from build123d import *

# Parameters (mm, degrees)
SKETCH1_R           = 70
BOSS_EXTRUDE2_DEPTH = 25
SKETCH3_R           = 70
BOSS_EXTRUDE3_DEPTH = 10
SKETCH4_R           = 3
CUT_EXTRUDE1_DEPTH  = 4
SKETCH5_R           = 23.5
CUT_EXTRUDE2_DEPTH  = 7
SKETCH6_R           = 1.5
CUT_EXTRUDE3_DEPTH  = 7
SKETCH7_R           = 22
CUT_EXTRUDE4_DEPTH  = 7
SKETCH8_R           = 70
CUT_EXTRUDE5_DEPTH  = 3
SKETCH9_R           = 1.425
CUT_EXTRUDE6_DEPTH  = 20


with BuildPart() as part:
    # Sketch1 → Boss-Extrude2 (new body)
    with BuildSketch(Plane.XY):
        Circle(SKETCH1_R)
        with BuildLine():
            ThreePointArc((5.084181722, 54.049826689), (0, 56.5), (-5.084181722, 54.049826689))
            ThreePointArc((-5.084181722, 54.049826689), (-14.092268161, 47.993857843), (-24.944456649, 48.218323814))
            ThreePointArc((-24.944456649, 48.218323814), (-30.546206186, 47.530824605), (-33.49862832, 42.720891489))
            ThreePointArc((-33.49862832, 42.720891489), (-37.802608913, 32.756147086), (-47.053406284, 27.077843822))
            ThreePointArc((-47.053406284, 27.077843822), (-51.394207738, 23.470948235), (-51.277497116, 17.828375092))
            ThreePointArc((-51.277497116, 17.828375092), (-49.510888436, 7.118591073), (-54.223231887, -2.659660261))
            ThreePointArc((-54.223231887, -2.659660261), (-55.924911466, -8.040788362), (-52.776122888, -12.724524427))
            ThreePointArc((-52.776122888, -12.724524427), (-45.499810707, -20.779067307), (-44.177564489, -31.552741003))
            ThreePointArc((-44.177564489, -31.552741003), (-42.699850951, -36.999631468), (-37.51870254, -39.237477348))
            ThreePointArc((-37.51870254, -39.237477348), (-27.042864565, -42.079518636), (-20.105832509, -50.428049418))
            ThreePointArc((-20.105832509, -50.428049418), (-15.917889462, -54.211353009), (-10.349359231, -53.29280845))
            ThreePointArc((-10.349359231, -53.29280845), (0, -50.020020118), (10.349359231, -53.29280845))
            ThreePointArc((10.349359231, -53.29280845), (15.917889462, -54.211353009), (20.105832509, -50.428049418))
            ThreePointArc((20.105832509, -50.428049418), (27.042864565, -42.079518636), (37.51870254, -39.237477348))
            ThreePointArc((37.51870254, -39.237477348), (42.699850951, -36.999631468), (44.177564489, -31.552741003))
            ThreePointArc((44.177564489, -31.552741003), (45.499810707, -20.779067307), (52.776122888, -12.724524427))
            ThreePointArc((52.776122888, -12.724524427), (55.924911466, -8.040788362), (54.223231887, -2.659660261))
            ThreePointArc((54.223231887, -2.659660261), (49.510888436, 7.118591073), (51.277497116, 17.828375092))
            ThreePointArc((51.277497116, 17.828375092), (51.394207738, 23.470948235), (47.053406284, 27.077843822))
            ThreePointArc((47.053406284, 27.077843822), (37.802608913, 32.756147086), (33.49862832, 42.720891489))
            ThreePointArc((33.49862832, 42.720891489), (30.546206186, 47.530824605), (24.944456649, 48.218323814))
            ThreePointArc((24.944456649, 48.218323814), (14.092268161, 47.993857843), (5.084181722, 54.049826689))
        make_face(mode=Mode.SUBTRACT)
    extrude(amount=BOSS_EXTRUDE2_DEPTH)

    # Sketch3 → Boss-Extrude3 (add)
    with BuildSketch(Plane.XY.offset(25)):
        Circle(SKETCH3_R)
    extrude(amount=BOSS_EXTRUDE3_DEPTH)

    # Sketch4 → Cut-Extrude1 (cut)
    with BuildSketch(Plane(origin=(0, 0, 25), x_dir=(-1, 0, 0), z_dir=(0, 0, -1))):
        with Locations((0, 50)):
            Circle(SKETCH4_R)
        with Locations((27.032040873, 42.062676642)):
            Circle(SKETCH4_R)
        with Locations((45.481599768, 20.77075065)):
            Circle(SKETCH4_R)
        with Locations((49.491072094, -7.115741914)):
            Circle(SKETCH4_R)
        with Locations((37.787478718, -32.743036697)):
            Circle(SKETCH4_R)
        with Locations((14.086627842, -47.974648681)):
            Circle(SKETCH4_R)
        with Locations((-14.086627842, -47.974648681)):
            Circle(SKETCH4_R)
        with Locations((-37.787478718, -32.743036697)):
            Circle(SKETCH4_R)
        with Locations((-49.491072094, -7.115741914)):
            Circle(SKETCH4_R)
        with Locations((-45.481599768, 20.77075065)):
            Circle(SKETCH4_R)
        with Locations((-27.032040873, 42.062676642)):
            Circle(SKETCH4_R)
    extrude(amount=-CUT_EXTRUDE1_DEPTH, mode=Mode.SUBTRACT)

    # Sketch5 → Cut-Extrude2 (cut)
    with BuildSketch(Plane(origin=(0, 0, 25), x_dir=(-1, 0, 0), z_dir=(0, 0, -1))):
        Circle(SKETCH5_R)
    extrude(amount=-CUT_EXTRUDE2_DEPTH, mode=Mode.SUBTRACT)

    # Sketch6 → Cut-Extrude3 (cut)
    with BuildSketch(Plane(origin=(0, 0, 29), x_dir=(-1, 0, 0), z_dir=(0, 0, -1))):
        with Locations((0, 50)):
            Circle(SKETCH6_R)
        with Locations((27.032040873, 42.062676642)):
            Circle(SKETCH6_R)
        with Locations((45.481599768, 20.77075065)):
            Circle(SKETCH6_R)
        with Locations((49.491072094, -7.115741914)):
            Circle(SKETCH6_R)
        with Locations((37.787478718, -32.743036697)):
            Circle(SKETCH6_R)
        with Locations((14.086627842, -47.974648681)):
            Circle(SKETCH6_R)
        with Locations((-14.086627842, -47.974648681)):
            Circle(SKETCH6_R)
        with Locations((-37.787478718, -32.743036697)):
            Circle(SKETCH6_R)
        with Locations((-49.491072094, -7.115741914)):
            Circle(SKETCH6_R)
        with Locations((-45.481599768, 20.77075065)):
            Circle(SKETCH6_R)
        with Locations((-27.032040873, 42.062676642)):
            Circle(SKETCH6_R)
    extrude(amount=-CUT_EXTRUDE3_DEPTH, mode=Mode.SUBTRACT)

    # Sketch7 → Cut-Extrude4 (cut)
    with BuildSketch(Plane(origin=(0, 0, 32), x_dir=(-1, 0, 0), z_dir=(0, 0, -1))):
        Circle(SKETCH7_R)
    extrude(amount=-CUT_EXTRUDE4_DEPTH, mode=Mode.SUBTRACT)

    # Sketch8 → Cut-Extrude5 (cut)
    with BuildSketch(Plane(origin=(0, 0, 0), x_dir=(-1, 0, 0), z_dir=(0, 0, -1))):
        Circle(SKETCH8_R)
    extrude(amount=-CUT_EXTRUDE5_DEPTH, mode=Mode.SUBTRACT)

    # Sketch9 → Cut-Extrude6 (cut)
    with BuildSketch(Plane(origin=(0, 0, 3), x_dir=(-1, 0, 0), z_dir=(0, 0, -1))):
        with Locations((0, 64)):
            Circle(SKETCH9_R)
        with Locations((55.425625842, 32)):
            Circle(SKETCH9_R)
        with Locations((55.425625842, -32)):
            Circle(SKETCH9_R)
        with Locations((0, -64)):
            Circle(SKETCH9_R)
        with Locations((-55.425625842, -32)):
            Circle(SKETCH9_R)
        with Locations((-55.425625842, 32)):
            Circle(SKETCH9_R)
    extrude(amount=-CUT_EXTRUDE6_DEPTH, mode=Mode.SUBTRACT)


solid = part.part
For this review, take the finished solid that the model builds, in its own axes (mm). Give positions to 0.01 mm unless a question says otherwise; leave off trailing zeros. Loops run counter-clockwise (first coordinate to the right, second up) from the corner with the lowest first, then second, coordinate; pieces in that order, holes last. Notation, with made-up numbers: M 88,-31 L 140,-31 A28 cw 140,3 Z; hole C -29,58 d6. An arc over 180 degrees is marked long. Answer as a JSON object with one key per item and string values. Group by question number.
Q1. Insertion check: P1, Ø0.9, axis at x = -55.5, y = 32.5, coming from the -Z side; P2, Ø1.5, axis at y = 16, z = 8.5, coming from the -X side; P3, Ø3, axis at y = 37.5, z = 9, coming from the -X side. Each pin has a flat end and moves straight along its axis. Give the tip position at first contact, or say it passes through.
Q2. For probe 1 along Y at (x, z) = (0, 27.75); probe 2 along Y at (x, z) = (46, 19.5); probe 3 along X at (y, z) = (29, 16), list the stretches that pass through material, from the lowest coordinate up. Write a range as [from, to].
Q3. Add section B-B on z = 9. Give the number of separate pieces and of enclosed holes in the cut face, and give its area (3 significant figures).
Q4. Add section A-A on y = 3.5. Give the boundary of the cut face in (x, z), and give its area (3 significant figures).
Q5. Mouldability with a two-part tool opening along Y and no side actions: class faces 1 (the flat face through (-17, -15, 35)), 2 (the cylindrical face through (-55.55, -42.594, 18.776)), 3 (the cylindrical face through (30.61, 47.49, 13.85)) as +Y half, -Y half, draft (parallel to the pull), parting line (faces both ways), or undercut.
Q6. Add section C-C on y = -17.5. Give the boundary of the cut face in (x, z), and give its area (3 significant figures).
Checked values:
{
 "1": {"P1": "z = 23", "P2": "x = -68.32", "P3": "x = -60.03"},
 "2": {"probe 1": "[-70, -23.5], [23.5, 47], [53, 70]", "probe 2": "[-52.76, -19.77], [27.37, 52.76]", "probe 3": "[-63.71, -42.33], [42.33, 63.71]"},
 "3": {"separate pieces": "1", "enclosed holes": "7", "area": "6,580 mm²"},
 "4": {"outline": "M -69.91,3 L -50.42,3 L -50.42,25 L -23.24,25 L -23.24,32 L -21.72,32 L -21.72,35 L -69.91,35 Z; M 21.72,32 L 23.24,32 L 23.24,25 L 50.42,25 L 50.42,3 L 69.91,3 L 69.91,35 L 21.72,35 Z", "area": "1,800 mm²"},
 "5": {"face 1": "draft", "face 2": "parting line", "face 3": "undercut"},
 "6": {"outline": "M -67.78,3 L -47.44,3 L -47.44,25 L -15.68,25 L -15.68,32 L -13.33,32 L -13.33,35 L -67.78,35 Z; M 13.33,32 L 15.68,32 L 15.68,25 L 47.44,25 L 47.44,3 L 67.78,3 L 67.78,35 L 13.33,35 Z", "area": "1,950 mm²"}
}
